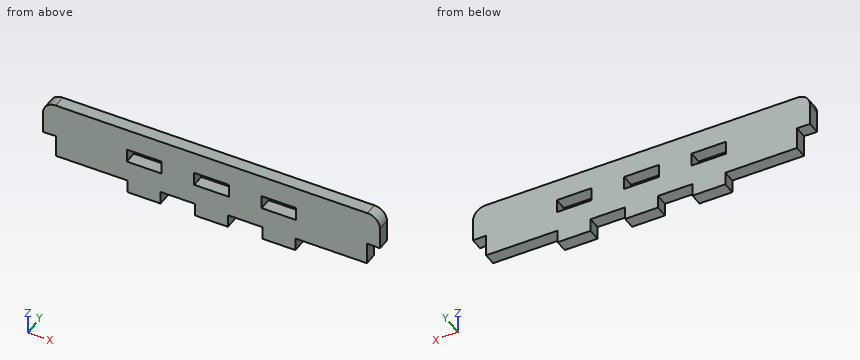
from build123d import *

# Parameters (mm, degrees)
SKETCH1_W           = 80
SKETCH1_H           = 16.5
BOSS_EXTRUDE1_DEPTH = 3
SKETCH3_W           = 8.2
SKETCH3_H           = 3.2
CUT_EXTRUDE1_DEPTH  = 4
FILLET1_R           = 3


with BuildPart() as part:
    # Sketch1 → Boss-Extrude1 (new body)
    with BuildSketch(Plane(origin=(0, 0, 0), x_dir=(1, 0, 0), z_dir=(0, 1, 0))):
        with Locations((40, -8.25)):
            Rectangle(SKETCH1_W, SKETCH1_H)
    extrude(amount=-BOSS_EXTRUDE1_DEPTH)

    # Sketch3 → Cut-Extrude1 (cut, through all)
    with BuildSketch(Plane(origin=(0, 0, 0), x_dir=(1, 0, 0), z_dir=(0, 1, 0))):
        with Locations((24, -9.7)):
            Rectangle(SKETCH3_W, SKETCH3_H)
        with Locations((40, -9.7)):
            Rectangle(SKETCH3_W, SKETCH3_H)
        with Locations((32, -1.5)):
            Rectangle(SKETCH3_W, SKETCH3_H)
        with Locations((56, -9.7)):
            Rectangle(SKETCH3_W, SKETCH3_H)
        with Locations((48, -1.5)):
            Rectangle(SKETCH3_W, SKETCH3_H)
        Polygon((76.9, -3.1), (76.9, -8.351680555), (80.1, -8.298347221), (80.1, 0.1), (59.9, 0.1), (59.9, -3.1), align=None)
        Polygon((-0.1, -8.298347221), (3.1, -8.351680555), (3.1, -3.1), (20.1, -3.1), (20.1, 0.1), (-0.1, 0.1), align=None)
    extrude(amount=-CUT_EXTRUDE1_DEPTH, mode=Mode.SUBTRACT)

    # Fillet1
    fillet1_edges = [part.edges().sort_by_distance(p)[0] for p in [
        (80, -1.5, 16.5),
        (0, -1.5, 16.5),
    ]]
    fillet(fillet1_edges, radius=FILLET1_R)


solid = part.part
Here's how the part is built. I have some questions about the finished solid (model axes, mm). Coordinates: 2 decimals unless noted, no trailing zeros. Order: outer loops, then holes, each group sorted by start corner. A loop starts at its lowest first (then second) coordinate and runs counter-clockwise, first axis right, second up.
Item 1: If we section it at D-D on z = 5.75: List the corners of the cut face in (x, y) for me, plus the area to 3 significant figures.
Result sheet:
outline: (3.1, -3) - (76.9, -3) - (76.9, 0) - (3.1, 0) - close
area: 221 mm2
Item 2: If we section it at A-A on z = 1.5: List the corners of the cut face in (x, y) for me.
Result sheet:
outline: (20.1, -3) - (27.9, -3) - (27.9, 0) - (20.1, 0) - close; (36.1, -3) - (43.9, -3) - (43.9, 0) - (36.1, 0) - close; (52.1, -3) - (59.9, -3) - (59.9, 0) - (52.1, 0) - close
Item 3: For P1, Ø1.5, axis at y = -1.5, z = 2, coming from the -X side; P2, Ø1.5, axis at y = -1.5, z = 5, coming from the -X side; P3, Ø0.9, axis at x = 8.5, y = -2, coming from the -Z side, each with a flat end and sliding along its axis, tell me the tip position at first contact or that it passes through.
Result sheet:
P1: stops at x = 20.1
P2: stops at x = 3.1
P3: stops at z = 3.1
Item 4: If we section it at B-B on x = 59: List the corners of the cut face in (y, z) for me, plus the area to 3 significant figures.
Result sheet:
outline: (-3, 0) - (0, 0) - (0, 8.1) - (-3, 8.1) - close; (-3, 11.3) - (0, 11.3) - (0, 16.5) - (-3, 16.5) - close
area: 39.9 mm2
Item 5: I need wall thicknesses on line 1 (X direction, y = -0.75, z = 10.5); line 2 (X direction, y = -2.35, z = 1.5); line 3 (Z direction, x = 25, y = -2.45). Which ranges of each line are inside material? Lowest first, please.
Result sheet:
line 1: x = 0 to 19.9, 28.1 to 35.9, 44.1 to 51.9, 60.1 to 80
line 2: x = 20.1 to 27.9, 36.1 to 43.9, 52.1 to 59.9
line 3: z = 0 to 8.1, 11.3 to 16.5
Item 6: If we section it at C-C on y = -0.6: State how many separate pieces and enclosed holes the cut face has, plus the area to 3 significant figures.
Result sheet:
separate pieces: 1
enclosed holes: 3
area: 1,030 mm2
